Part print with two shaded views. Sizes in mm from the minimum x, y, z corner. A direction names the side the tool comes from. Coordinates: 2 decimals unless noted, no trailing zeros. Order: outer loops, then holes, each group sorted by start corner. A loop starts at its lowest first (then second) coordinate and runs counter-clockwise, first axis right, second up. Notation, with made-up numbers: (31, -1) - (90, -1) arc R4 ccw to (90, 4) - close; hole circle Ø6 at (72, 45). An arc over 180 degrees is marked (long way). Write each question's results on one line, items separated by ' | '. Start each with the question number.
Q1. Which spindle directions (+Z, -Z, +X, -X, +Y, -Y) get a long thin tool onto all of the face, cutting with end or side? Do the marked faces 1 and 2. Say none if no direction does.
Q2. Band-saw the part on C-C, the plane z = 12.75. Write the cut outline in (x, y).
Q3. Pull direction Z, two halves, no side cores. Call the marked faces 3, 4, 5 and 6: released by +Z, released by -Z, zero draft, split by the parting line, or undercut.
Q4. Pin check, flat tips, straight feed: P1, Ø10.5, axis at x = 12, y = 13, coming from the +Z side; P2, Ø10, axis at y = 8.5, z = 9, coming from the -X side; P3, Ø12, axis at x = 17, z = 12, coming from the +Y side; P4, Ø4, axis at x = 10, z = 15, coming from the -Y side. Stop position of each tip, or through.
Q5. Band-saw the part on A-A, the plane x = 10. Write the cut outline in (y, z).
Q6. Band-saw the part on B-B, the plane y = 2.25. Write the cut outline in (x, z).
Q7. Wall check: probe 1 along Z at (x, y) = (10, 4.25); probe 2 along Z at (x, y) = (7, 10); probe 3 along Y at (x, z) = (18.25, 8.75). Give the ranges that are in metal, low to high.
Q8. Band-saw the part on D-D, the plane y = 9. Write the cut outline in (x, z), then the cut area to 3 significant figures.
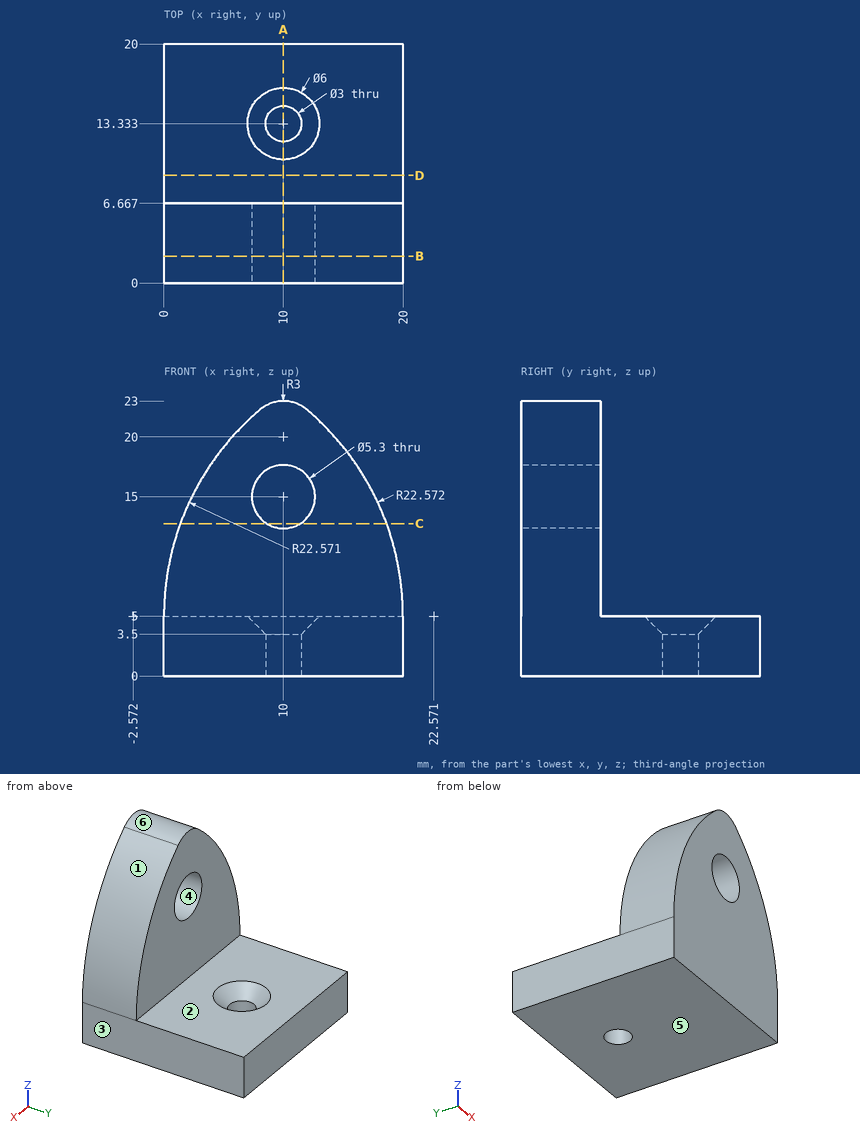
Results below:
1) face 1: +Z, +X, +Y, -Y | face 2: +Z, +X, -X, +Y
2) outline: (1.37, 0) - (8.6, 0) - (8.6, 6.67) - (1.37, 6.67) - close; (11.4, 0) - (18.63, 0) - (18.63, 6.67) - (11.4, 6.67) - close
3) face 3: zero draft | face 4: undercut | face 5: released by -Z | face 6: released by +Z
4) P1: stops at z = 5 | P2: stops at x = 0 | P3: stops at y = 6.67 | P4: passes through
5) outline: (0, 0) - (11.83, 0) - (11.83, 3.5) - (10.33, 5) - (6.67, 5) - (6.67, 12.35) - (0, 12.35) - close; (0, 17.65) - (6.67, 17.65) - (6.67, 23) - (0, 23) - close; (14.83, 0) - (20, 0) - (20, 5) - (16.33, 5) - (14.83, 3.5) - close
6) outline: (0, 0) - (20, 0) - (20, 5) arc R22.57 ccw to (11.93, 22.3) arc R3 ccw to (8.07, 22.3) arc R22.57 ccw to (0, 5) - close; hole circle Ø5.3 at (10, 15)
7) probe 1: z = 0 to 12.35, 17.65 to 23 | probe 2: z = 0 to 5 | probe 3: y = 0 to 6.67
8) outline: (0, 0) - (20, 0) - (20, 5) - (0, 5) - close | area: 100 mm²
